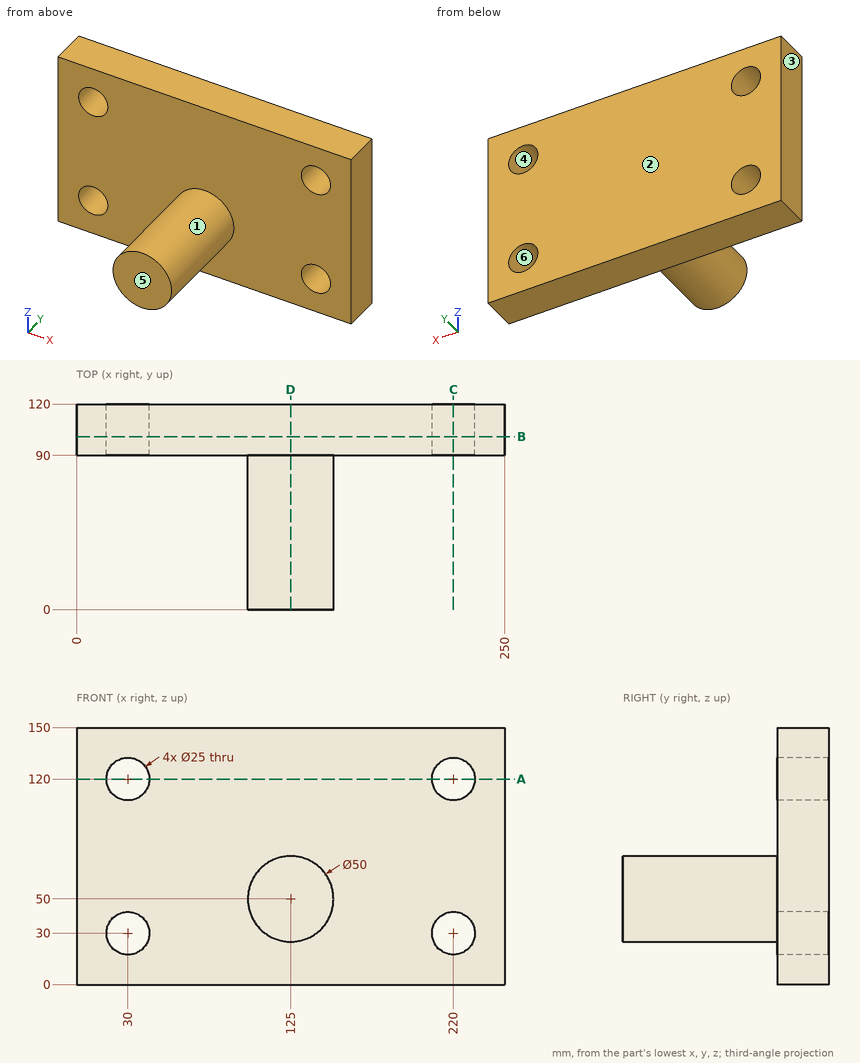
For this review, use the dimensioned drawing (mm, ordinates from the lowest corner) and the shaded views. A direction names the side the tool comes from. Coordinates: 2 decimals unless noted, no trailing zeros. Loops run counter-clockwise (first coordinate to the right, second up) from the corner with the lowest first, then second, coordinate; pieces in that order, holes last. Notation, with made-up numbers: (-25, 4) -> (26, 4) arc R15 cw to (26, 20) -> close; hole circle Ø10 at (5, 42). An arc over 180 degrees is marked (long way). Use a Markdown table: item, result. Add a question column.
1. Add section D-D on x = 125. Write out the cut boundary in (y, z), plus the area to 3 significant figures.
2. To check wall thickness, follow line 1 (Z direction, x = 220, y = 108.5); line 2 (X direction, y = 108, z = 120); line 3 (X direction, y = 90.5, z = 123). State the ranges of each line that lie inside material, in increasing order.
3. Add section B-B on y = 101. Write out the cut boundary in (x, z).
4. Add section A-A on z = 120. Write out the cut boundary in (x, y), plus the area to 3 significant figures.
5. Machinability: for the marked faces 1 and 2, which of the approach directions +Z, -Z, +X, -X, +Y, -Y give a long, thin tool a straight path to every point of the face, cutting with its end or side? Answer none if there is none.
6. Draft analysis for pull direction X (two halves, no side actions). For the marked faces 3, 4, 5 and 6, state which applies: pulls with the +X half, pulls with the -X half, needs draft (parallel to the pull), parting line crosses it, or undercut.
7. Add section C-C on x = 220. Write out the cut boundary in (y, z).
8. Clearance check with flat-ended pins moving along their axes: pin 1 Ø2 at (x, y) = (134.5, 54) entering from +Z; pin 2 Ø12 at (y, z) = (35.5, 76.5) entering from -X; pin 3 Ø22.5 at (x, z) = (220, 30) entering from +Y. State where each tip first meets the part, or that it passes through.
Returned:
| question | item | result |
|---|---|---|
| 1 | outline | (0, 25) -> (90, 25) -> (90, 0) -> (120, 0) -> (120, 150) -> (90, 150) -> (90, 75) -> (0, 75) -> close |
| 1 | area | 9,000 mm² |
| 2 | line 1 | z = 0 to 17.5, 42.5 to 107.5, 132.5 to 150 |
| 2 | line 2 | x = 0 to 17.5, 42.5 to 207.5, 232.5 to 250 |
| 2 | line 3 | x = 0 to 17.87, 42.13 to 207.87, 232.13 to 250 |
| 3 | outline | (0, 0) -> (250, 0) -> (250, 150) -> (0, 150) -> close; hole circle Ø25 at (30, 30); hole circle Ø25 at (30, 120); hole circle Ø25 at (220, 30); hole circle Ø25 at (220, 120) |
| 4 | outline | (0, 90) -> (17.5, 90) -> (17.5, 120) -> (0, 120) -> close; (42.5, 90) -> (207.5, 90) -> (207.5, 120) -> (42.5, 120) -> close; (232.5, 90) -> (250, 90) -> (250, 120) -> (232.5, 120) -> close |
| 4 | area | 6,000 mm² |
| 5 | face 1 | -Y |
| 5 | face 2 | +Z, -Z, +X, -X, +Y |
| 6 | face 3 | pulls with the -X half |
| 6 | face 4 | undercut |
| 6 | face 5 | needs draft |
| 6 | face 6 | undercut |
| 7 | outline | (90, 0) -> (120, 0) -> (120, 17.5) -> (90, 17.5) -> close; (90, 42.5) -> (120, 42.5) -> (120, 107.5) -> (90, 107.5) -> close; (90, 132.5) -> (120, 132.5) -> (120, 150) -> (90, 150) -> close |
| 8 | pin 1 | stops at z = 73.51 |
| 8 | pin 2 | stops at x = 110.69 |
| 8 | pin 3 | passes through |
